Part model, mm, in its own coordinate system. A direction names the side the tool comes from. Give positions to 0.01 mm unless a question says otherwise; leave off trailing zeros. Order: outer loops, then holes, each group sorted by start corner. A loop starts at its lowest first (then second) coordinate and runs counter-clockwise, first axis right, second up.
from build123d import *

# Parameters (mm, degrees)
BOSS_EXTRUDE2_DEPTH = 11.43
SKETCH7_OUTSIDE_W   = 59.664
SKETCH7_OUTSIDE_H   = 63.75
SKETCH7_OUTSIDE_R   = 13.208
CUT_EXTRUDE1_DEPTH  = 11.43
CUT_EXTRUDE1_DRAFT  = -45
SKETCH9_R           = 6.35
BOSS_EXTRUDE6_DEPTH = 114.3
CHAMFER3_SIZE       = 1.016


with BuildPart() as part:
    # Sketch5 → Boss-Extrude2 (new body)
    with BuildSketch(Plane(origin=(0, 0, 0), x_dir=(1, 0, 0), z_dir=(0, 1, 0))):
        Polygon((13.208, -7.625642355), (13.208, 7.625642355), (0, 15.251284711), (-13.208, 7.625642355), (-13.208, -7.625642355), (0, -15.251284711), align=None)
    extrude(amount=BOSS_EXTRUDE2_DEPTH)


with BuildPart() as cut_extrude1_tool:
    # Sketch7 outside → Cut-Extrude1 (with draft: the straight prism first)
    with BuildSketch(Plane(origin=(0, 11.43, 0), x_dir=(1, 0, 0), z_dir=(0, 1, 0))):
        Rectangle(SKETCH7_OUTSIDE_W, SKETCH7_OUTSIDE_H)
        Circle(SKETCH7_OUTSIDE_R, mode=Mode.SUBTRACT)
    extrude(amount=-CUT_EXTRUDE1_DEPTH)
    # Cut-Extrude1: the draft: its side faces are tilted about the plane it starts from
    cut_extrude1_sides = [cut_extrude1_tool.faces().sort_by_distance(p)[0] for p in [
        (0, 5.715, 31.875),
        (29.832, 5.715, 0),
        (0, 5.715, -31.875),
        (-29.832, 5.715, 0),
        (-13.208, 5.715, 0),
    ]]
    draft(cut_extrude1_sides, Plane(origin=(0, 11.43, 0), x_dir=(1, 0, 0), z_dir=(0, 1, 0)), CUT_EXTRUDE1_DRAFT)


with BuildPart() as part_1:
    add(part.part)

    # Cut-Extrude1: cut by cut_extrude1_tool
    add(cut_extrude1_tool.part, mode=Mode.SUBTRACT)

    # Sketch9 → Boss-Extrude6 (add)
    with BuildSketch(Plane(origin=(0, 0, 0), x_dir=(-1, 0, 0), z_dir=(0, -1, 0))):
        with Locations(Location((0, 0, 0), (0, 0, 90))):
            Circle(SKETCH9_R)
    extrude(amount=BOSS_EXTRUDE6_DEPTH)

    # Chamfer3
    chamfer3_edges = [part_1.edges().sort_by_distance(p)[0] for p in [
        (0, -114.3, 6.35),
    ]]
    chamfer(chamfer3_edges, length=CHAMFER3_SIZE)


solid = part_1.part
Item 1: Drop flat-ended pins along their axis: P1, Ø5, axis at x = 4.5, y = -61.5, coming from the -Z side; P2, Ø2, axis at x = 1.5, y = -63, coming from the +Z side; P3, Ø1, axis at x = -5.5, y = -73, coming from the -Z side. Give the stop position or say it passes through.
Item 2: Drill centre lines: probe 1 along Y at (x, z) = (10, -8); probe 2 along X at (y, z) = (-89, -0.5); probe 3 along Z at (x, y) = (1, -28). Where is each one in solid material? Low to high.
Item 3: Which spindle directions (+Z, -Z, +X, -X, +Y, -Y) get a long thin tool onto all of the face, cutting with end or side? Do faces 1 (the face through (0, 0, 7)), 2 (the face through (-11.844, 10.943, -6.877)). Say none if no direction does.
Item 4: Band-saw the part on A-A on y = -57. List the corners of the cut face in (x, z), plus the area to 3 significant figures.
Working result:
1. P1: stops at z = -6.03
1. P2: stops at z = 6.33
1. P3: stops at z = -3.91
2. probe 1: y = 0 to 11.43
2. probe 2: x = -6.33 to 6.33
2. probe 3: z = -6.27 to 6.27
3. face 1: -Y
3. face 2: -Z, -X, +Y
4. outline: circle Ø12.7 at (0, 0)
4. area: 127 mm2
